The model under review builds one solid part; all positions refer to its coordinate system, in mm. A direction names the side the tool comes from. Give positions to 0.01 mm unless a question says otherwise; leave off trailing zeros. Loops run counter-clockwise (first coordinate to the right, second up) from the corner with the lowest first, then second, coordinate; pieces in that order, holes last. Notation, with made-up numbers: M -3.75,-32 L 4.25,-32 A26 cw 4.25,1 Z; hole C 83.25,-10 d3. An arc over 180 degrees is marked long. Return JSON: item names as keys, results as strings.
```python
from build123d import *

# Parameters (mm, degrees)
SKETCH1_R                = 14
SKETCH1_R_2              = 11
BOSS_EXTRUDE1_DEPTH      = 8
SKETCH2_W                = 3.5
SKETCH2_H                = 8
SKETCH4_R                = 14
SKETCH4_R_2              = 7
BOSS_EXTRUDE2_DEPTH      = 2
BOSS_EXTRUDE3_DEPTH      = 2
BOSS_EXTRUDE3_DEPTH_BACK = 2
SKETCH5_R                = 0.75


with BuildPart() as part:
    # Sketch1 → Boss-Extrude1 (new body)
    with BuildSketch(Plane(origin=(0, 0, 0), x_dir=(0, 0, -1), z_dir=(1, 0, 0))):
        Circle(SKETCH1_R)
        Circle(SKETCH1_R_2, mode=Mode.SUBTRACT)
    extrude(amount=BOSS_EXTRUDE1_DEPTH)

    # Sketch2 → Revolve1 (revolve)
    with BuildSketch(Plane(origin=(4, 0, 0), x_dir=(0, 0, -1), z_dir=(1, 0, 0))):
        with Locations((1.75, 16)):
            Rectangle(SKETCH2_W, SKETCH2_H)
    revolve1 = revolve(axis=Axis((4, 12, 0), (0, 1, 0)))

    # Sketch3 → Revolve2 (revolve)
    with BuildSketch(Plane(origin=(4, 0, 0), x_dir=(0, 0, -1), z_dir=(1, 0, 0))):
        with BuildLine():
            Line((0, 14), (0, 26))
            ThreePointArc((0, 26), (6, 20), (0, 14))
        make_face()
    revolve2 = revolve(axis=Axis((4, 14, 0), (0, 1, 0)))

    # Mirror1: Revolve1, Revolve2 across plane
    add(revolve1.mirror(Plane.ZX))
    add(revolve2.mirror(Plane.ZX))

    # Sketch4 → Boss-Extrude2 (add)
    with BuildSketch(Plane(origin=(8, 0, 0), x_dir=(0, 0, -1), z_dir=(1, 0, 0))):
        Circle(SKETCH4_R)
        Circle(SKETCH4_R_2, mode=Mode.SUBTRACT)
    extrude(amount=BOSS_EXTRUDE2_DEPTH)

    # Sketch5 → Boss-Extrude3 (add, two sides: drawn at the far end of the back side and taken through both)
    with BuildSketch(Plane(origin=(0, 0, 0), x_dir=(1, 0, 0), z_dir=(0, 1, 0)).offset(-BOSS_EXTRUDE3_DEPTH_BACK)):
        with BuildLine():
            Line((10, 13), (0, 13))
            Line((0, 13), (-7.508861075, 27.122113749))
            ThreePointArc((-7.508861075, 27.122113749), (-7.405739907, 31.0601523), (-3.977070704, 33))
            Line((-3.977070704, 33), (-3.934896023, 33))
            ThreePointArc((-3.934896023, 33), (-1.940550712, 32.467360203), (-0.477339242, 31.01129339))
            Line((-0.477339242, 31.01129339), (10, 13))
        make_face()
        with Locations(Location((-3.977070704, 29, 0), (0, 0, 270))):
            Circle(SKETCH5_R, mode=Mode.SUBTRACT)
    extrude(amount=BOSS_EXTRUDE3_DEPTH + BOSS_EXTRUDE3_DEPTH_BACK)


solid = part.part
```
1) Consider section D-D on x = 5.5. Write out the cut boundary in (y, z), then the cut area to 3 significant figures.
From the geometry:
{"outline": "M -15.13,-3.16 L -13.64,-3.16 A14 ccw -2,-13.86 L -2,-20.74 L 2,-20.74 L 2,-13.86 A14 ccw 13.64,-3.16 L 15.13,-3.16 A5.81 ccw long 15.13,3.16 L 13.64,3.16 A14 ccw -13.64,3.16 L -15.13,3.16 A5.81 ccw long Z; hole C 0,0 d22", "area": "483 mm²"}
2) Tool access review of faces 1 (the face through (5.341, -14.525, -3.233)), 2 (the face through (3.94, -10.74, 2.38)), 3 (the face through (-3.7, -0.03, -19.96)): name each direction out of +Z, -Z, +X, -X, +Y, -Y from which nothing blocks a thin tool from reaching the whole face with its end or side.
From the geometry:
{"face 1": "none", "face 2": "-X", "face 3": "+Z, -X, +Y, -Y"}
3) The part is to be moulded in two halves that separate along Y. For faces 4 (the face through (-1, 2, -23)), 5 (the face through (10, 3.3, 6.4)), 6 (the face through (0, -11.3, 0.1)), 7 (the face through (4.9, -12.4, -6.5)), say which applies: released by +Y, released by -Y, zero draft, split by the parting line, or undercut.
From the geometry:
{"face 4": "released by +Y", "face 5": "zero draft", "face 6": "undercut", "face 7": "undercut"}
4) Wall thickness on L1, parallel to Y at x = 8.85, z = 0; L2, parallel to Y at x = 0.25, z = -3.5; L3, parallel to Z at x = 0.25, y = -4.5: over which ranges is each line inside the solid? List them lowest first. Write a range as from..to.
From the geometry:
{"L1": "-23.53..-16.47, -14..-7, 7..14, 16.47..23.53", "L2": "-23.11..-16.89, -13.56..-10.43, 10.43..13.56, 16.89..23.11", "L3": "-13.26..-10.04, 10.04..13.26"}
5) Consider section B-B on y = 0. Write out the cut boundary in (x, z), then the cut area to 3 significant figures.
From the geometry:
{"outline": "M -7.51,-27.12 A4 ccw -3.98,-33 L -3.93,-33 A4 ccw -0.48,-31.01 L 9.42,-14 L 10,-14 L 10,-7 L 8,-7 L 8,-11 L 0,-11 L 0,-13 Z; M 0,11 L 8,11 L 8,7 L 10,7 L 10,14 L 0,14 Z; hole C -3.98,-29 d1.5", "area": "244 mm²"}
6) Insertion check: pin 1 (8 mm diameter, centred on y = -7.5, z = -10, fed in from -X); pin 2 (10 mm diameter, centred on y = -3, z = -21.5, fed in from -X); pin 3 (0.9 mm diameter, centred on x = -3.98, z = -29, fed in from -Y); pin 4 (8.5 mm diameter, centred on x = 4.5, z = -22.5, fed in from +Y). Each pin has a flat end and moves straight along its axis. Give the tip position at first contact, or say it passes through.
From the geometry:
{"pin 1": "x = 0", "pin 2": "x = -7.12", "pin 3": "through", "pin 4": "y = 2"}
7) Consider section C-C on x = 2.25. Write out the cut boundary in (y, z), then the cut area to 3 significant figures.
From the geometry:
{"outline": "M -15.13,-3.03 L -13.67,-3.03 A14 ccw -2,-13.86 L -2,-26.32 L 2,-26.32 L 2,-13.86 A14 ccw 13.67,-3.03 L 15.13,-3.03 A5.74 ccw long 15.13,3.03 L 13.67,3.03 A14 ccw -13.67,3.03 L -15.13,3.03 A5.74 ccw long Z; hole C 0,0 d22", "area": "500 mm²"}
8) Consider section A-A on z = 0. Write out the cut boundary in (x, y).
From the geometry:
{"outline": "M 0,-14 L 0.5,-14 L 0.5,-15.13 A6 ccw long 7.5,-15.13 L 7.5,-14 L 10,-14 L 10,-7 L 8,-7 L 8,-11 L 0,-11 Z; M 0,11 L 8,11 L 8,7 L 10,7 L 10,14 L 7.5,14 L 7.5,15.13 A6 ccw long 0.5,15.13 L 0.5,14 L 0,14 Z"}
